from build123d import *

# Parameters (mm, degrees)
SKETCH1_W           = 0.25
SKETCH1_H           = 1
SKETCH1_W_2         = 22.96
SKETCH1_H_2         = 22.96
SKETCH1_W_3         = 22.45
SKETCH1_H_3         = 22.45
SKETCH1_W_4         = 9.5
SKETCH1_H_4         = 0.255
SKETCH1_W_5         = 3.45
SKETCH1_H_5         = 3.45
SKETCH1_R           = 0.975
SKETCH1_W_6         = 1
SKETCH1_H_6         = 0.25
SKETCH1_W_7         = 4.9
SKETCH1_H_7         = 4.9
BOSS_EXTRUDE5_DEPTH = 0.2


with BuildPart() as part:
    # Sketch1 → Boss-Extrude5 (new body)
    # profile 1 of 18: a face of its own
    with BuildSketch(Plane(origin=(0, 0, 0), x_dir=(1, 0, 0), z_dir=(0, 1, 0))):
        with Locations((-11.605, -1.95)):
            Rectangle(SKETCH1_W, SKETCH1_H)
    # profile 2 of 18: a face of its own
    with BuildSketch(Plane(origin=(0, 0, 0), x_dir=(1, 0, 0), z_dir=(0, 1, 0))):
        with Locations((-11.605, 1.95)):
            Rectangle(SKETCH1_W, SKETCH1_H)
    # profile 3 of 18: a face of its own
    with BuildSketch(Plane(origin=(0, 0, 0), x_dir=(1, 0, 0), z_dir=(0, 1, 0))):
        Rectangle(SKETCH1_W_2, SKETCH1_H_2)
        Rectangle(SKETCH1_W_3, SKETCH1_H_3, mode=Mode.SUBTRACT)
    # profile 4 of 18: a face of its own
    with BuildSketch(Plane(origin=(0, 0, 0), x_dir=(1, 0, 0), z_dir=(0, 1, 0))):
        with Locations((-6.475, 1.5975)):
            Rectangle(SKETCH1_W_4, SKETCH1_H_4)
    # profile 5 of 18: a face of its own
    with BuildSketch(Plane(origin=(0, 0, 0), x_dir=(1, 0, 0), z_dir=(0, 1, 0))):
        with Locations((-6.475, -1.5975)):
            Rectangle(SKETCH1_W_4, SKETCH1_H_4)
    # profile 6 of 18: a face of its own
    with BuildSketch(Plane(origin=(0, 0, 0), x_dir=(1, 0, 0), z_dir=(0, 1, 0))):
        with Locations((6.475, 1.5975)):
            Rectangle(SKETCH1_W_4, SKETCH1_H_4)
    # profile 7 of 18: a face of its own
    with BuildSketch(Plane(origin=(0, 0, 0), x_dir=(1, 0, 0), z_dir=(0, 1, 0))):
        with Locations((6.475, -1.5975)):
            Rectangle(SKETCH1_W_4, SKETCH1_H_4)
    # profile 8 of 18: a face of its own
    with BuildSketch(Plane(origin=(0, 0, 0), x_dir=(1, 0, 0), z_dir=(0, 1, 0))):
        with Locations((11.605, 1.95)):
            Rectangle(SKETCH1_W, SKETCH1_H)
    # profile 9 of 18: a face of its own
    with BuildSketch(Plane(origin=(0, 0, 0), x_dir=(1, 0, 0), z_dir=(0, 1, 0))):
        with Locations((11.605, -1.95)):
            Rectangle(SKETCH1_W, SKETCH1_H)
    # profile 10 of 18: a face of its own
    with BuildSketch(Plane(origin=(0, 0, 0), x_dir=(1, 0, 0), z_dir=(0, 1, 0))):
        Rectangle(SKETCH1_W_5, SKETCH1_H_5)
        with Locations(Location((0, 0, 0), (0, 0, 270))):
            Circle(SKETCH1_R, mode=Mode.SUBTRACT)
    # profile 11 of 18: a face of its own
    with BuildSketch(Plane(origin=(0, 0, 0), x_dir=(1, 0, 0), z_dir=(0, 1, 0))):
        Polygon((-1.45, -11.73), (-2.45, -11.73), (-2.45, -11.98), (2.45, -11.98), (2.45, -11.73), (1.45, -11.73), align=None)
    # profile 12 of 18: a face of its own
    with BuildSketch(Plane(origin=(0, 0, 0), x_dir=(1, 0, 0), z_dir=(0, 1, 0))):
        with Locations((1.95, -11.605)):
            Rectangle(SKETCH1_W_6, SKETCH1_H_6)
    # profile 13 of 18: a face of its own
    with BuildSketch(Plane(origin=(0, 0, 0), x_dir=(1, 0, 0), z_dir=(0, 1, 0))):
        with Locations((-1.95, -11.605)):
            Rectangle(SKETCH1_W_6, SKETCH1_H_6)
    # profile 14 of 18: a face of its own
    with BuildSketch(Plane(origin=(0, 0, 0), x_dir=(1, 0, 0), z_dir=(0, 1, 0))):
        Polygon((11.98, 2.45), (11.73, 2.45), (11.73, 1.45), (11.73, -1.45), (11.73, -2.45), (11.98, -2.45), align=None)
    # profile 15 of 18: a face of its own
    with BuildSketch(Plane(origin=(0, 0, 0), x_dir=(1, 0, 0), z_dir=(0, 1, 0))):
        with Locations((1.95, 11.605)):
            Rectangle(SKETCH1_W_6, SKETCH1_H_6)
    # profile 16 of 18: a face of its own
    with BuildSketch(Plane(origin=(0, 0, 0), x_dir=(1, 0, 0), z_dir=(0, 1, 0))):
        with Locations((0, 11.855)):
            Rectangle(SKETCH1_W_7, SKETCH1_H_6)
    # profile 17 of 18: a face of its own
    with BuildSketch(Plane(origin=(0, 0, 0), x_dir=(1, 0, 0), z_dir=(0, 1, 0))):
        with Locations((-1.95, 11.605)):
            Rectangle(SKETCH1_W_6, SKETCH1_H_6)
    # profile 18 of 18: a face of its own
    with BuildSketch(Plane(origin=(0, 0, 0), x_dir=(1, 0, 0), z_dir=(0, 1, 0))):
        with Locations((-11.855, 0)):
            Rectangle(SKETCH1_W, SKETCH1_H_7)
    extrude(amount=BOSS_EXTRUDE5_DEPTH)


solid = part.part
CAD build for the part. Positions are in the model's coordinates, mm. Round coordinates to 2 decimals unless told otherwise and drop trailing zeros. Write each loop counter-clockwise with the first axis right and the second up, starting at its lowest first coordinate (ties: lowest second). Pieces come first, ordered by that corner, then holes. Notation, with made-up numbers: M 61.25,53.5 L 77.25,53.5 A16 cw 77.25,66.5 Z; hole C 70.5,81.5 d10. An arc over 180 degrees is marked long. Put each result on its own line as item: value. Start each with the question number.
1) Saw through at D-D, the plane x = 0. Write the cut outline in (y, z) (3 decimals), and give its area (3 significant figures).
2) Saw through at B-B, the plane z = 4. Write the cut outline in (x, y) (3 decimals).
3) Pin check, flat tip, straight feed: pin 1 Ø1 at (x, z) = (-1.5, 4) entering from -Y. Stop position of the tip, or through.
4) Saw through at A-A, the plane x = 4.75. Write the cut outline in (y, z) (3 decimals), and give its area (3 significant figures).
5) Drill centre lines: probe 1 along Z at (x, y) = (-2.5, 0.15) (3 decimals); probe 2 along X at (y, z) = (0.15, 0) (3 decimals); probe 3 along X at (y, z) = (0.15, 5.5) (3 decimals). Where is each one in solid material? Low to high. Write a range as [from, to].
6) Saw through at C-C, the plane z = 0. Write the cut outline in (x, y) (3 decimals).
Resolved:
1. outline: M 0,-11.98 L 0.2,-11.98 L 0.2,-11.73 L 0,-11.73 Z; M 0,-11.48 L 0.2,-11.48 L 0.2,-11.225 L 0,-11.225 Z; M 0,-1.725 L 0.2,-1.725 L 0.2,-0.975 L 0,-0.975 Z; M 0,0.975 L 0.2,0.975 L 0.2,1.725 L 0,1.725 Z; M 0,11.225 L 0.2,11.225 L 0.2,11.48 L 0,11.48 Z; M 0,11.73 L 0.2,11.73 L 0.2,11.98 L 0,11.98 Z
1. area: 0.502 mm²
2. outline: M -11.48,0 L -11.225,0 L -11.225,0.2 L -11.48,0.2 Z; M 11.225,0 L 11.48,0 L 11.48,0.2 L 11.225,0.2 Z
3. pin 1: through
4. outline: M 0,-11.48 L 0.2,-11.48 L 0.2,-11.225 L 0,-11.225 Z; M 0,-1.725 L 0.2,-1.725 L 0.2,-1.47 L 0,-1.47 Z; M 0,1.47 L 0.2,1.47 L 0.2,1.725 L 0,1.725 Z; M 0,11.225 L 0.2,11.225 L 0.2,11.48 L 0,11.48 Z
4. area: 0.204 mm²
5. probe 1: [-11.48, -11.225], [-1.725, -1.47], [1.47, 1.725], [11.225, 11.48]
5. probe 2: [-11.98, -11.73], [-11.48, -11.225], [-1.725, -0.975], [0.975, 1.725], [11.225, 11.48], [11.73, 11.98]
5. probe 3: [-11.48, -11.225], [11.225, 11.48]
6. outline: M -11.98,0 L -11.73,0 L -11.73,0.2 L -11.98,0.2 Z; M -11.48,0 L -11.225,0 L -11.225,0.2 L -11.48,0.2 Z; M -1.725,0 L -0.975,0 L -0.975,0.2 L -1.725,0.2 Z; M 0.975,0 L 1.725,0 L 1.725,0.2 L 0.975,0.2 Z; M 11.225,0 L 11.48,0 L 11.48,0.2 L 11.225,0.2 Z; M 11.73,0 L 11.98,0 L 11.98,0.2 L 11.73,0.2 Z
